Build history of the part. All positions in model axes, mm. Round coordinates to 2 decimals unless told otherwise and drop trailing zeros. Loops run counter-clockwise (first coordinate to the right, second up) from the corner with the lowest first, then second, coordinate; pieces in that order, holes last. Notation, with made-up numbers: M -10,21.25 L 15,21.25 A25 cw 15,60.25 Z; hole C 85.25,81 d4. An arc over 180 degrees is marked long. One line per item, written item: value.
```python
from build123d import *

# Parameters (mm, degrees)
BOX_W           = 120
BOX_H           = 100
BOX_DEPTH       = 30
SKETCH_W        = 114
SKETCH_H        = 94
POCKET_DEPTH    = 27
SKETCH001_W     = 114
SKETCH001_H     = 20
PAD_DEPTH       = 15
SKETCH002_W     = 114
SKETCH002_H     = 5
POCKET001_DEPTH = 10
SKETCH003_W     = 94
SKETCH003_H     = 20
POCKET002_DEPTH = 15
SKETCH008_R     = 1.43
POCKET005_DEPTH = 2.7
FILLET_R        = 5
SKETCH011_W     = 60
SKETCH011_H     = 40
POCKET008_DEPTH = 2


with BuildPart() as part:
    # Box → Box (new body)
    with BuildSketch(Plane.XY):
        with Locations((60, 50)):
            Rectangle(BOX_W, BOX_H)
    extrude(amount=BOX_DEPTH)

    # Sketch (on Face6 of BaseFeature) → Pocket (cut)
    with BuildSketch(Plane.XY.offset(30)):
        with Locations((60, 50)):
            Rectangle(SKETCH_W, SKETCH_H)
    extrude(amount=-POCKET_DEPTH, mode=Mode.SUBTRACT)

    # Sketch001 (on Face11 of Pocket) → Pad (join)
    with BuildSketch(Plane.XY.offset(3)):
        with Locations((60, 50)):
            Rectangle(SKETCH001_W, SKETCH001_H)
    extrude(amount=PAD_DEPTH)

    # Sketch002 (on Face13 of Pad) → Pocket001 (cut)
    with BuildSketch(Plane.XY.offset(18)):
        with Locations((60, 55)):
            Rectangle(SKETCH002_W, SKETCH002_H)
        with Locations((60, 45)):
            Rectangle(SKETCH002_W, SKETCH002_H)
    extrude(amount=-POCKET001_DEPTH, mode=Mode.SUBTRACT)

    # Sketch003 (on Face15 of Pocket001) → Pocket002 (cut)
    with BuildSketch(Plane.XY.offset(18)):
        with Locations((60, 50)):
            Rectangle(SKETCH003_W, SKETCH003_H)
    extrude(amount=-POCKET002_DEPTH, mode=Mode.SUBTRACT)

    # Sketch008 (on Face41 of Pocket002) → Pocket005 (cut)
    with BuildSketch(Plane.XY.offset(8)):
        with Locations((112, 45)):
            Circle(SKETCH008_R)
        with Locations((112, 55)):
            Circle(SKETCH008_R)
        with Locations((8, 45)):
            Circle(SKETCH008_R)
        with Locations((8, 55)):
            Circle(SKETCH008_R)
    extrude(amount=-POCKET005_DEPTH, mode=Mode.SUBTRACT)

    # Fillet
    fillet_edges = [part.edges().sort_by_distance(p)[0] for p in [
        (60, 0, 0),
        (60, 3, 3),
        (60, 97, 3),
        (60, 100, 0),
    ]]
    fillet(fillet_edges, radius=FILLET_R)

    # Sketch011 (on Face5 of Fillet) → Pocket008 (cut)
    with BuildSketch(Plane(origin=(0, 0, 0), x_dir=(1, 0, 0), z_dir=(0, 0, -1))):
        with Locations((60, -50)):
            Rectangle(SKETCH011_W, SKETCH011_H)
    extrude(amount=-POCKET008_DEPTH, mode=Mode.SUBTRACT)


solid = part.part
```
Item 1: Slice it at D-D, the plane y = 88. Give the cut face in (x, z).
Check values:
outline: M 0,0 L 120,0 L 120,30 L 117,30 L 117,3 L 3,3 L 3,30 L 0,30 Z
Item 2: Pull direction Y, two halves, no side cores. Call faces 1 (the face through (112, 59, 18)), 2 (the face through (59, 100, 17)), 3 (the face through (59, 0, 17)): pulls with the +Y half, pulls with the -Y half, needs draft (parallel to the pull), parting line crosses it, or undercut.
Check values:
face 1: undercut
face 2: pulls with the +Y half
face 3: pulls with the -Y half
Item 3: Drop flat-ended pins along their axis: P1, Ø1.5, axis at x = 110, y = 54.5, coming from the +Z side; P2, Ø8, axis at y = 19, z = 10.5, coming from the -X side; P3, Ø1.5, axis at x = 111.5, y = 45, coming from the +Z side; P4, Ø1.2, axis at x = 10, y = 59, coming from the +Z side. Give the stop position or say it passes through.
Check values:
P1: stops at z = 8
P2: stops at x = 0
P3: stops at z = 5.3
P4: stops at z = 18
Item 4: Slice it at A-A, the plane y = 45. Give the cut face in (x, z).
Check values:
outline: M 0,0 L 30,0 L 30,2 L 90,2 L 90,0 L 120,0 L 120,30 L 117,30 L 117,8 L 113.43,8 L 113.43,5.3 L 110.57,5.3 L 110.57,8 L 107,8 L 107,3 L 13,3 L 13,8 L 9.43,8 L 9.43,5.3 L 6.57,5.3 L 6.57,8 L 3,8 L 3,30 L 0,30 Z
Item 5: Wall check: line 1 along X through (y, z) = (6.5, 24.5); line 2 along Y through (x, z) = (44, 24.5); line 3 along Y through (x, z) = (112, 6.4). Give the ranges that are in metal, low to high.
Check values:
line 1: x = 0 to 3, 117 to 120
line 2: y = 0 to 3, 97 to 100
line 3: y = 0 to 3.26, 40 to 43.57, 46.43 to 53.57, 56.43 to 60, 96.74 to 100
Item 6: Slice it at C-C, the plane y = 34. Give the cut face in (x, z), and give its area (3 significant figures).
Check values:
outline: M 0,0 L 30,0 L 30,2 L 90,2 L 90,0 L 120,0 L 120,30 L 117,30 L 117,3 L 3,3 L 3,30 L 0,30 Z
area: 402 mm2
